Source: CAD feature listing. Evaluate the final solid. Frame: model axes, mm. Face numbers are marked on the shaded views. Round coordinates to 2 decimals unless told otherwise and drop trailing zeros. Order: outer loops, then holes, each group sorted by start corner. A loop starts at its lowest first (then second) coordinate and runs counter-clockwise, first axis right, second up. Notation, with made-up numbers: M 37,62.25 L 89,62.25 A19 cw 89,72.25 Z; hole C 50.25,47 d10. An arc over 180 degrees is marked long. Use one line per item in the form item = value. Start each with the question number.
Q1. Section A-A (x = 0). Return the cut outline in (y, z), plus the area to 3 significant figures.
Q2. Material intervals for probe 1 along Y at (x, z) = (0, 15); probe 2 along Y at (x, z) = (15, 14.5); probe 3 along Z at (x, y) = (-7.5, -10), sorted ascending.
Q3. Contact query for flat-ended pins moving along their axis: pin 1 (12 mm diameter, centred on y = -15.5, z = 17, fed in from +X); pin 2 (4.5 mm diameter, centred on x = -0.5, z = 5, fed in from +Y); pin 3 (4 mm diameter, centred on x = 0, y = 0, fed in from +Z); pin 4 (6 mm diameter, centred on y = -33, z = 12, fed in from +X). Output: stop coordinate, or through.
Q4. Pull-direction query (X, two-part tool) for the marked faces 1, 2 and 3; classes: pulls with the +X half, pulls with the -X half, needs draft (parallel to the pull), parting line crosses it, or undercut.
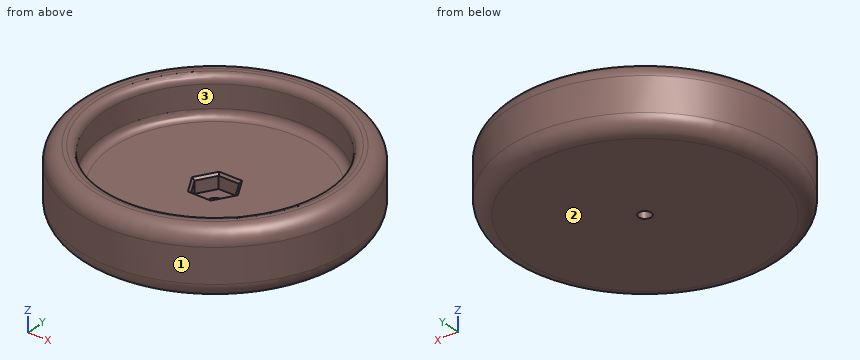
from build123d import *

# Parameters (mm, degrees)
SKETCH_R        = 46.0375
SKETCH_R_2      = 2.0955
PAD_DEPTH       = 21.59
SKETCH001_R     = 37.1475
POCKET_DEPTH    = 12.7
POCKET001_DEPTH = 4.826
FILLET_R        = 5.08
FILLET001_R     = 2.54
CHAMFER_SIZE    = 0.762


with BuildPart() as part:
    # Sketch → Pad (new body)
    with BuildSketch(Plane.XY):
        Circle(SKETCH_R)
        Circle(SKETCH_R_2, mode=Mode.SUBTRACT)
    extrude(amount=PAD_DEPTH)

    # Sketch001 (on Face4 of Pad) → Pocket (cut)
    with BuildSketch(Plane.XY.offset(21.59)):
        Circle(SKETCH001_R)
    extrude(amount=-POCKET_DEPTH, mode=Mode.SUBTRACT)

    # Sketch002 (on Face6 of Pocket) → Pocket001 (cut)
    with BuildSketch(Plane.XY.offset(8.89)):
        Polygon((6.928203, 0), (3.464102, 6), (-3.464102, 6), (-6.928203, 0), (-3.464102, -6), (3.464102, -6), align=None)
    extrude(amount=-POCKET001_DEPTH, mode=Mode.SUBTRACT)

    # Fillet
    fillet_edges = [part.edges().sort_by_distance(p)[0] for p in [
        (-46.0375, 0, 21.59),
        (-46.0375, 0, 0),
    ]]
    fillet(fillet_edges, radius=FILLET_R)

    # Fillet001
    fillet001_edges = [part.edges().sort_by_distance(p)[0] for p in [
        (-37.1475, 0, 21.59),
        (-37.1475, 0, 8.89),
    ]]
    fillet(fillet001_edges, radius=FILLET001_R)

    # Chamfer
    chamfer_edges = [part.edges().sort_by_distance(p)[0] for p in [
        (-5.196152, 3, 8.89),
        (-5.196152, -3, 8.89),
        (0, -6, 8.89),
        (5.196152, -3, 8.89),
        (5.196152, 3, 8.89),
        (0, 6, 8.89),
    ]]
    chamfer(chamfer_edges, length=CHAMFER_SIZE)


solid = part.part
Results list:
q1.outline = M -46.04,5.08 A5.08 ccw -40.96,0 L -2.1,0 L -2.1,4.06 L -6,4.06 L -6,8.13 L -6.76,8.89 L -34.61,8.89 A2.54 cw -37.15,11.43 L -37.15,19.05 A2.54 ccw -39.69,21.59 L -40.96,21.59 A5.08 ccw -46.04,16.51 Z; M 2.1,0 L 40.96,0 A5.08 ccw 46.04,5.08 L 46.04,16.51 A5.08 ccw 40.96,21.59 L 39.69,21.59 A2.54 ccw 37.15,19.05 L 37.15,11.43 A2.54 cw 34.61,8.89 L 6.76,8.89 L 6,8.13 L 6,4.06 L 2.1,4.06 Z
q1.area = 947 mm2
q2.probe_1 = -46.04 to -37.15, 37.15 to 46.04
q2.probe_2 = -43.53 to -33.98, 33.98 to 43.53
q2.probe_3 = 0 to 8.89
q3.pin_1 = 45.04
q3.pin_2 = 46.04
q3.pin_3 = through
q3.pin_4 = 34.92
q4.face_1 = parting line crosses it
q4.face_2 = needs draft
q4.face_3 = undercut
